Verification items for this drawing (mm, ordinates from the low corner). A direction names the side the tool comes from. Coordinates: 2 decimals unless noted, no trailing zeros. Write each loop counter-clockwise with the first axis right and the second up, starting at its lowest first coordinate (ties: lowest second). Pieces come first, ordered by that corner, then holes. Notation, with made-up numbers: (68.25, -24.75) -> (121.25, -24.75) arc R18 ccw to (121.25, 5.25) -> close; hole circle Ø10 at (22, 78). An arc over 180 degrees is marked (long way). Answer as CSV lines item,"result".
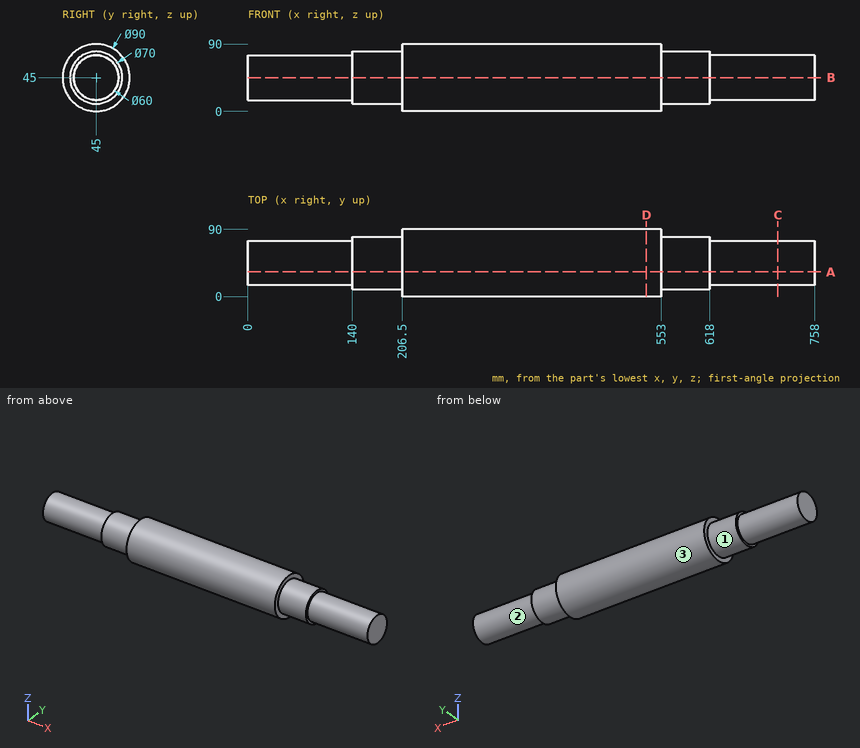
Item 1: Thickness scan on probe 1 along X at (y, z) = (47, 77.5); probe 2 along X at (y, z) = (78.5, 15); probe 3 along Z at (x, y) = (691, 17.5). Record the ranges inside material, lowest first.
Responses:
probe 1,"x = 140 to 618"
probe 2,"x = 206.5 to 553"
probe 3,"z = 33.01 to 56.99"
Item 2: Cross-section at B-B, the plane z = 45. Record the cut outline in (x, y), plus the area to 3 significant figures.
Responses:
outline,"(0, 15) -> (140, 15) -> (140, 10) -> (206.5, 10) -> (206.5, 0) -> (553, 0) -> (553, 10) -> (618, 10) -> (618, 15) -> (758, 15) -> (758, 75) -> (618, 75) -> (618, 80) -> (553, 80) -> (553, 90) -> (206.5, 90) -> (206.5, 80) -> (140, 80) -> (140, 75) -> (0, 75) -> close"
area,"57,200 mm2"
Item 3: Cross-section at D-D, the plane x = 533. Record the cut outline in (y, z), plus the area to 3 significant figures.
Responses:
outline,"circle Ø90 at (45, 45)"
area,"6,360 mm2"
Item 4: Depth check by flat-ended pin: pin 1 Ø1 at (x, y) = (593, 16.5) entering from +Z; pin 2 Ø2 at (x, y) = (240.5, 34) entering from -Z; pin 3 Ø3 at (x, y) = (348, 61) entering from -Z. Enter the tip coordinate at first touch or a pass-through.
Responses:
pin 1,"stops at z = 66"
pin 2,"stops at z = 1.13"
pin 3,"stops at z = 2.4"
Item 5: Cross-section at A-A, the plane y = 33. Record the cut outline in (x, z).
Responses:
outline,"(0, 17.5) -> (140, 17.5) -> (140, 12.12) -> (206.5, 12.12) -> (206.5, 1.63) -> (553, 1.63) -> (553, 12.12) -> (618, 12.12) -> (618, 17.5) -> (758, 17.5) -> (758, 72.5) -> (618, 72.5) -> (618, 77.88) -> (553, 77.88) -> (553, 88.37) -> (206.5, 88.37) -> (206.5, 77.88) -> (140, 77.88) -> (140, 72.5) -> (0, 72.5) -> close"
Item 6: Cross-section at C-C, the plane x = 709. Record the cut outline in (y, z), plus the area to 3 significant figures.
Responses:
outline,"circle Ø60 at (45, 45)"
area,"2,830 mm2"
Item 7: Set-up check for the marked faces 1, 2 and 3: record each of +Z, -Z, +X, -X, +Y, -Y from which the full face is reachable in a straight line by a thin tool's end or side.
Responses:
face 1,"-X"
face 2,"+X"
face 3,"+X, -X"
